CAD build for the part. Positions are in the model's coordinates, mm. Face numbers are marked on the shaded views. A direction names the side the tool comes from. Coordinates: 2 decimals unless noted, no trailing zeros. Order: outer loops, then holes, each group sorted by start corner. A loop starts at its lowest first (then second) coordinate and runs counter-clockwise, first axis right, second up. Notation, with made-up numbers: (-12, 58) -> (-4, 58) arc R11 cw to (-4, 65) -> close; hole circle Ø10 at (27, 64.5). An arc over 180 degrees is marked (long way). Use one line per item in the form item = value. Start each with the question number.
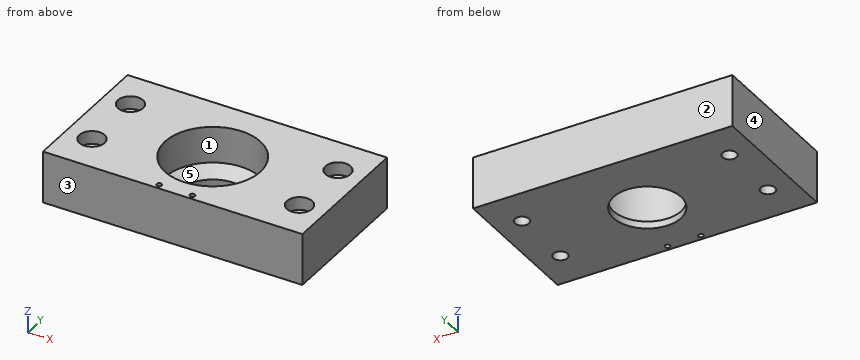
from build123d import *

# Parameters (mm, degrees)
F0_W           = 100
F0_H           = 55
F1_DEPTH       = 20
F3_D           = 26
F4_D           = 36.8
F4_DEPTH       = 14
F4_TIP         = 11.0558353901
F6_D           = 2
F8_D           = 5.5
F8_CBORE_D     = 9.75
F8_CBORE_DEPTH = 5


with BuildPart() as f1:
    # F0 (on Top) → F1 (new body)
    with BuildSketch(Plane.XY):
        with Locations((-2.2873312235, 1.0893514007)):
            Rectangle(F0_W, F0_H)
    extrude(amount=F1_DEPTH)

    # F3 (through all)
    with Locations(Plane.XY.offset(20)):
        with Locations((-2.2873312235, -0.4106485993)):
            Hole(F3_D / 2)

    # F4
    with Locations(Plane.XY.offset(20)):
        with Locations((-2.2873312235, -0.4106485993)):
            Hole(F4_D / 2, depth=F4_DEPTH)
            with Locations((0, 0, -(F4_DEPTH + F4_TIP / 2))):  # 118° drill point
                Cone(0, F4_D / 2, F4_TIP, mode=Mode.SUBTRACT)

    # F6 (through all)
    with Locations(Plane.XY.offset(20)):
        with Locations((-8.6873312235, -24.4106485993), (4.1126687765, -24.4106485993)):
            Hole(F6_D / 2)

    # F8 (through all)
    with Locations(Plane.XY.offset(20)):
        with Locations((-42.2873312235, 13.5893514007), (-42.2873312235, -11.4106485993), (37.7126687765, -11.4106485993), (37.7126687765, 13.5893514007)):
            CounterBoreHole(F8_D / 2, F8_CBORE_D / 2, F8_CBORE_DEPTH)


solid = f1.part
1) Cut at A-A on z = 17. Give the cut face in (x, y) (3 decimals).
2) Drop a flat-ended pin along its axis: P1, Ø5, axis at x = -42.5, y = -11, coming from the +Z side. Give the stop position or say it passes through.
3) Two-plate mould, pull along Y, no slides. Class the marked faces 3, 4 and 5: released by +Y, released by -Y, zero draft, split by the parting line, or undercut.
4) Cut at B-B on z = 7.5. Give the cut face in (x, y), then the cut area to 3 significant figures.
5) 3-axis set-ups, long thin cutter, end or side, ignore diameter. For the marked faces 1 and 2: which of +Z, -Z, +X, -X, +Y, -Y reach the whole face in a straight line?
6) Probe L1, parallel to Y at x = 36, z = 6.25; L2, parallel to X at y = -10, z = 1.5; L3, parallel to X at y = 14, z = 15.5 (3 decimals). List the from-to ranges inside material, lowest first.
Values follow:
q1.outline = (-52.287, -26.411) -> (47.713, -26.411) -> (47.713, 28.589) -> (-52.287, 28.589) -> close; hole circle Ø9.75 at (-42.287, -11.411); hole circle Ø9.75 at (-42.287, 13.589); hole circle Ø36.8 at (-2.287, -0.411); hole circle Ø2 at (-8.687, -24.411); hole circle Ø2 at (4.113, -24.411); hole circle Ø9.75 at (37.713, -11.411); hole circle Ø9.75 at (37.713, 13.589)
q2.P1 = 15
q3.face_3 = released by -Y
q3.face_4 = zero draft
q3.face_5 = undercut
q4.outline = (-52.29, -26.41) -> (47.71, -26.41) -> (47.71, 28.59) -> (-52.29, 28.59) -> close; hole circle Ø5.5 at (-42.29, -11.41); hole circle Ø5.5 at (-42.29, 13.59); hole circle Ø36.8 at (-2.29, -0.41); hole circle Ø2 at (-8.69, -24.41); hole circle Ø2 at (4.11, -24.41); hole circle Ø5.5 at (37.71, -11.41); hole circle Ø5.5 at (37.71, 13.59)
q4.area = 4,340 mm^2
q5.face_1 = +Z
q5.face_2 = +Z, -Z, +X, -X, +Y
q6.L1 = -26.41 to -13.56, -9.26 to 11.44, 15.74 to 28.59
q6.L2 = -52.29 to -44.65, -39.93 to -11.06, 6.49 to 35.35, 40.07 to 47.71
q6.L3 = -52.287 to -47.145, -37.43 to -13.728, 9.154 to 32.855, 42.57 to 47.713
